The listing builds one solid part. Answer for the finished solid, in the listing's coordinates (mm). Face numbers are marked on the shaded views. A direction names the side the tool comes from. Coordinates: 2 decimals unless noted, no trailing zeros. Order: outer loops, then holes, each group sorted by start corner. A loop starts at its lowest first (then second) coordinate and runs counter-clockwise, first axis right, second up. Notation, with made-up numbers: (84, 0) -> (118, 0) arc R33 ccw to (118, 30) -> close; hole circle Ø5 at (66, 5). An arc over 180 degrees is marked (long way). One line per question, with ' | ' between items.
from build123d import *

# Parameters (mm, degrees)
F1_DEPTH      = 10
F1_DEPTH_BACK = 10
F5_DEPTH      = 28
F8_D          = 2.8
F8_ON_F2_D    = 2.8
F9_D          = 3.4
F9_ON_F2_D    = 3.4
F10_DEPTH     = 10
F11_F1_R      = 3
F11_F2_R      = 3
F11_F3_R      = 3
F11_F4_R      = 3
F11_F5_R      = 3
F11_F6_R      = 3
F12_DEPTH     = 10


with BuildPart() as f1:
    # F0 (on Front) → F1 (new body, two sides)
    with BuildSketch(Plane.XZ) as f1_sk:
        with BuildLine():
            Line((15, 17), (0, 17))
            Line((0, 17), (0, 11.81))
            ThreePointArc((0, 11.81), (8.3509310858, 8.3509310858), (11.81, 0))
            ThreePointArc((11.81, 0), (8.3509310858, -8.3509310858), (0, -11.81))
            Line((0, -11.81), (0, -17))
            Line((0, -17), (15, -17))
            Line((15, -17), (15, 17))
        make_face()
    extrude(amount=F1_DEPTH)
    extrude(f1_sk.sketch, amount=-F1_DEPTH_BACK)

    # F2 (on face) → F3 (revolve, cut)
    with BuildSketch(Plane(origin=(0, 0, 0), x_dir=(0, -1, 0), z_dir=(-1, 0, 0))):
        with BuildLine():
            Line((-1.25, -11.81), (1.25, -11.81))
            ThreePointArc((1.25, -11.81), (0, -10.56), (-1.25, -11.81))
        make_face()
        with BuildLine():
            ThreePointArc((-1.25, -11.81), (0, -13.06), (1.25, -11.81))
            Line((1.25, -11.81), (-1.25, -11.81))
        make_face()
    revolve(axis=Axis((0, 0, 0), (0, -1, 0)), mode=Mode.SUBTRACT)

    # F4 (on face) → F5 (join)
    with BuildSketch(Plane(origin=(0, 10, 0), x_dir=(-1, 0, 0), z_dir=(0, 1, 0))):
        with BuildLine():
            Line((0, -11.81), (0, 11.81))
            ThreePointArc((0, 11.81), (-11.81, 0), (0, -11.81))
        make_face()
        with BuildLine():
            Line((0, 17), (-15, 17))
            Line((-15, 17), (-15, -17))
            Line((-15, -17), (0, -17))
            Line((0, -17), (0, -11.81))
            ThreePointArc((0, -11.81), (-11.81, 0), (0, 11.81))
            Line((0, 11.81), (0, 17))
        make_face()
    extrude(amount=F5_DEPTH)

    # F6: union 

    # F8 (through all)
    with Locations(Plane(origin=(0, 0, 0), x_dir=(0, -1, 0), z_dir=(-1, 0, 0))):
        with Locations((-13.5, 14)):
            Hole(F8_D / 2)

    # F8 on F2 (through all)
    with Locations(Plane(origin=(0, 0, 0), x_dir=(0, -1, 0), z_dir=(-1, 0, 0))):
        with Locations((6.5, -14)):
            Hole(F8_ON_F2_D / 2)

    # F9 (through all)
    with Locations(Plane(origin=(0, 0, 0), x_dir=(0, -1, 0), z_dir=(-1, 0, 0))):
        with Locations((-13.5, -14)):
            Hole(F9_D / 2)

    # F9 on F2 (through all)
    with Locations(Plane(origin=(0, 0, 0), x_dir=(0, -1, 0), z_dir=(-1, 0, 0))):
        with Locations((6.5, 14)):
            Hole(F9_ON_F2_D / 2)

    # F7 (on face) → F10 (cut)
    with BuildSketch(Plane(origin=(0, 0, 0), x_dir=(0, -1, 0), z_dir=(-1, 0, 0))):
        with BuildLine():
            Line((-38, 11.75), (-38, -11.75))
            Line((-38, -11.75), (-25.1889491158, -11.75))
            ThreePointArc((-25.1889491158, -11.75), (-35.81, 0), (-25.1889491158, 11.75))
            Line((-25.1889491158, 11.75), (-38, 11.75))
        make_face()
        with BuildLine():
            ThreePointArc((-25.1889491158, 11.75), (-35.81, 0), (-25.1889491158, -11.75))
            Line((-25.1889491158, -11.75), (-24, -11.75))
            Line((-24, -11.75), (-24, 11.75))
            Line((-24, 11.75), (-25.1889491158, 11.75))
        make_face()
    extrude(amount=-F10_DEPTH, mode=Mode.SUBTRACT)

    # F11: fillet of radius 3 on 6 edges, made by hand

    # F11_f1
    f11_f1_edges = [f1.edges().sort_by_distance(p)[0] for p in [
        (5, 38, 11.75),
    ]]
    fillet(f11_f1_edges, radius=F11_F1_R)

    # F11_f2
    f11_f2_edges = [f1.edges().sort_by_distance(p)[0] for p in [
        (5, 38, -11.75),
    ]]
    fillet(f11_f2_edges, radius=F11_F2_R)

    # F11_f3
    f11_f3_edges = [f1.edges().sort_by_distance(p)[0] for p in [
        (7.5, -10, 17),
    ]]
    fillet(f11_f3_edges, radius=F11_F3_R)

    # F11_f4
    f11_f4_edges = [f1.edges().sort_by_distance(p)[0] for p in [
        (7.5, 38, 17),
    ]]
    fillet(f11_f4_edges, radius=F11_F4_R)

    # F11_f5
    f11_f5_edges = [f1.edges().sort_by_distance(p)[0] for p in [
        (7.5, -10, -17),
    ]]
    fillet(f11_f5_edges, radius=F11_F5_R)

    # F11_f6
    f11_f6_edges = [f1.edges().sort_by_distance(p)[0] for p in [
        (7.5, 38, -17),
    ]]
    fillet(f11_f6_edges, radius=F11_F6_R)

    # F7 (on face) → F12 (cut)
    with BuildSketch(Plane(origin=(0, 0, 0), x_dir=(0, -1, 0), z_dir=(-1, 0, 0))):
        with BuildLine():
            Line((-24, -11.75), (-25.1889491158, -11.75))
            ThreePointArc((-25.1889491158, -11.75), (-16.0805741704, -8.7612096499), (-12.19, 0))
            ThreePointArc((-12.19, 0), (-16.0805741704, 8.7612096499), (-25.1889491158, 11.75))
            Line((-25.1889491158, 11.75), (-24, 11.75))
            Line((-24, 11.75), (-24, -11.75))
        make_face()
    extrude(amount=-F12_DEPTH, mode=Mode.SUBTRACT)


solid = f1.part
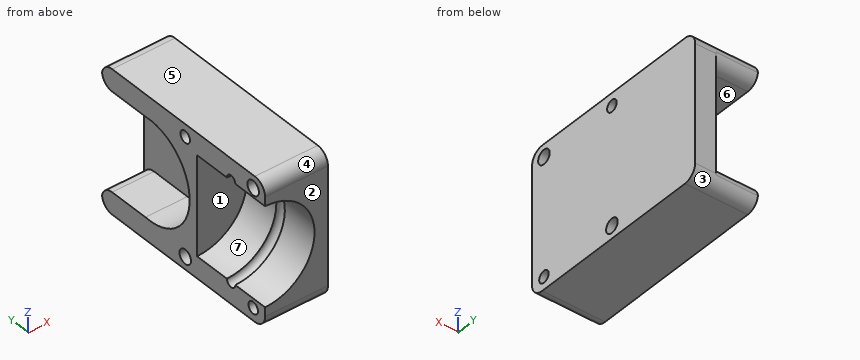
Item 1: Section C-C, the plane y = 33 is taken. Give the vertices of the cut face in (x, z), plus the area to 3 significant figures.
Computed values:
outline: (0, -17) -> (15, -17) -> (15, 17) -> (0, 17) -> (0, 11.75) -> (10, 11.75) -> (10, -11.75) -> (0, -11.75) -> close | area: 275 mm^2
Item 2: Section D-D, the plane x = 5.25 is taken. Count the separate pieces of the cut face and the enclosed holes in it, plus the area to 3 significant figures.
Computed values:
separate pieces: 1 | enclosed holes: 4 | area: 613 mm^2
Item 3: Determine the mould class of the marked faces 1, 2, 3 and 4 for opening direction Z: pulls with the +Z half, pulls with the -Z half, needs draft (parallel to the pull), parting line crosses it, or undercut.
Computed values:
face 1: undercut | face 2: needs draft | face 3: pulls with the -Z half | face 4: pulls with the +Z half
Item 4: For the marked faces 5, 6 and 7, determine the directions among +Z, -Z, +X, -X, +Y, -Y from which every point of the face is accessible in a straight line to the end or side of a thin tool.
Computed values:
face 5: +Z, +X, -X, +Y, -Y | face 6: -X, +Y | face 7: -X, -Y
Item 5: Find the intervals of material crossed by L1, parallel to Z at x = 4.5, y = 24; L2, parallel to Y at x = 10.25, z = -14.5; L3, parallel to X at y = 25, z = -10, in increasing order.
Computed values:
L1: z = -17 to -11.81, 11.81 to 17 | L2: y = -9.96 to -7.81, -5.19 to 11.88, 15.12 to 37.96 | L3: x = 10 to 15
Item 6: Each of these flat-tipped pins is pushed along its axis until it touches: pin 1 Ø3 at (x, z) = (9.5, 6) entering from +Y; pin 2 Ø8 at (y, z) = (4.5, -3.5) entering from -X; pin 3 Ø4 at (y, z) = (24, 1) entering from -X; pin 4 Ø3.5 at (x, z) = (5.5, -5) entering from -Y. Where does it stop, or does it pass through?
Computed values:
pin 1: stops at y = 38 | pin 2: stops at x = 9.12 | pin 3: stops at x = 10 | pin 4: stops at y = 10
Item 7: Section B-B, the plane z = 0 is taken. Give the vertices of the cut face in (x, y), plus the area to 3 significant figures.
Computed values:
outline: (0, 10) -> (11.81, 10) -> (11.81, 1.25) arc R1.25 cw to (11.81, -1.25) -> (11.81, -10) -> (15, -10) -> (15, 38) -> (10, 38) -> (10, 12.19) -> (0, 12.19) -> close | area: 223 mm^2
Item 8: Section A-A, the plane y = -6.5 is taken. Give the vertices of the cut face in (x, z), plus the area to 3 significant figures.
Computed values:
outline: (0, -17) -> (15, -17) -> (15, -15.4) -> (0, -15.4) -> close; (0, -12.6) -> (15, -12.6) -> (15, 12.3) -> (0, 12.3) -> (0, 11.81) arc R11.81 cw to (0, -11.81) -> close; (0, 15.7) -> (15, 15.7) -> (15, 17) -> (0, 17) -> close | area: 198 mm^2
